The model under review builds one solid part; all positions refer to its coordinate system, in mm. Face numbers are marked on the shaded views. A direction names the side the tool comes from. Round coordinates to 2 decimals unless told otherwise and drop trailing zeros. Loops run counter-clockwise (first coordinate to the right, second up) from the corner with the lowest first, then second, coordinate; pieces in that order, holes last. Notation, with made-up numbers: (34.25, 73.25) -> (90.25, 73.25) arc R22 ccw to (90.25, 85.25) -> close; hole circle Ø9 at (36.5, 29). An arc over 180 degrees is marked (long way). Use a Markdown table: item, result. Add a question column.
1) Mouldability with a two-part tool opening along Y and no side actions: class the marked faces 1, 2 and 3 as released by +Y, released by -Y, zero draft, split by the parting line, or undercut.
2) Wall thickness on probe 1 along X at (y, z) = (-15.5, 5.5); probe 2 along X at (y, z) = (-9, 6.5); probe 3 along X at (y, z) = (10, 3.5): over which ranges is each line inside the solid? List them lowest first.
3) Insertion check: pin 1 (1 mm diameter, centred on x = -9.5, z = 1.5, fed in from -Y); pin 2 (2 mm diameter, centred on y = 23.5, z = 3, fed in from +X); pin 3 (6 mm diameter, centred on x = 11.14, y = 11.14, fed in from +Z); pin 4 (2 mm diameter, centred on x = -20.67, y = 7.52, fed in from +Z). Each pin has a flat end and moves straight along its axis. Give the tip position at first contact, or say it passes through.
4) Consider section A-A on z = 7. State how many separate pieces and enclosed holes the cut face has, plus the area to 3 significant figures.
5) For the marked faces 4 and 5, list the 3-axis set-ups (+Z, -Z, +X, -X, +Y, -Y) from which the entire face can be reached by the end or side of a thin tool; tool diameter is ignored.
6) Consider section B-B on y = 20. Give the boundary of the cut face in (x, z), plus the area to 3 significant figures.
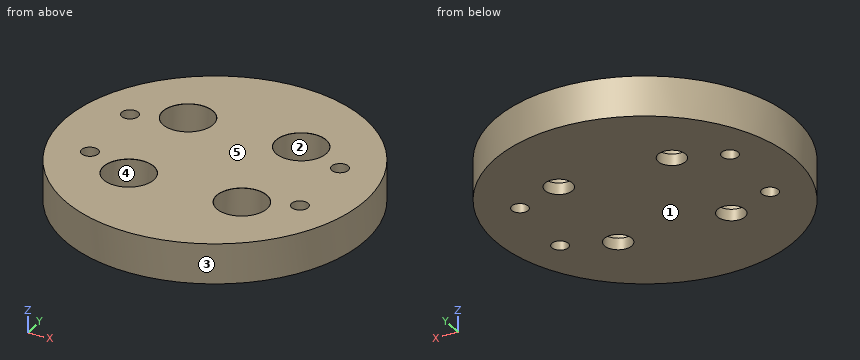
from build123d import *

# Parameters (mm, degrees)
SKETCH_1_R               = 30
EXTRUDE_1_DEPTH          = 8
PATTERN_CIRCULAR_1_COUNT = 4
HOLE_WIZARD_M4_1_D       = 3.3


with BuildPart() as part:
    # 草图1 → 凸台-拉伸1 (new body)
    with BuildSketch(Plane.XY):
        Circle(SKETCH_1_R)
    extrude(amount=EXTRUDE_1_DEPTH)

    # 草图7 → 打孔尺寸(%根据)内六角圆柱头螺钉的类型1 (revolve, cut)
    with BuildSketch(Plane(origin=(11.136931804, -11.136931804, 8), x_dir=(0, -1, 0), z_dir=(1, 0, 0))):
        Polygon((0, 0), (0, 8), (2.75, 8), (2.75, 5.7), (5, 5.7), (5, 0.025), (5.025, 0), align=None)
    hole_wizard_1 = revolve(axis=Axis((11.136931804, -11.136931804, 14.35), (0, 0, -1)), mode=Mode.SUBTRACT)

    # 阵列(圆周)1: 打孔尺寸(%根据)内六角圆柱头螺钉的类型1 ×4 about axis
    pattern_circular_1_axis = Axis((0, 0, 0), (0, 0, 1))
    for i in range(1, PATTERN_CIRCULAR_1_COUNT):
        add(hole_wizard_1.rotate(pattern_circular_1_axis, i * 360 / PATTERN_CIRCULAR_1_COUNT), mode=Mode.SUBTRACT)

    # M4 螺纹孔1 (through all)
    with Locations(Plane.XY.offset(8)):
        with Locations((20.673237657, 7.524443153), (20.673237657, -7.524443153), (-20.673237657, 7.524443153), (-20.673237657, -7.524443153)):
            Hole(HOLE_WIZARD_M4_1_D / 2)


solid = part.part
Result set:
| question | item | result |
|---|---|---|
| 1 | face 1 | zero draft |
| 1 | face 2 | undercut |
| 1 | face 3 | split by the parting line |
| 2 | probe 1 | -25.69 to -13.58, -8.69 to 8.69, 13.58 to 25.69 |
| 2 | probe 2 | -28.62 to -21.41, -19.93 to -15.66, -6.62 to 6.62, 15.66 to 19.93, 21.41 to 28.62 |
| 2 | probe 3 | -28.28 to -16.01, -6.27 to 6.27, 16.01 to 28.28 |
| 3 | pin 1 | y = -28.62 |
| 3 | pin 2 | x = 19.84 |
| 3 | pin 3 | z = 2.3 |
| 3 | pin 4 | through |
| 4 | separate pieces | 1 |
| 4 | enclosed holes | 8 |
| 4 | area | 2,480 mm2 |
| 5 | face 4 | +Z |
| 5 | face 5 | +Z, +X, -X, +Y, -Y |
| 6 | outline | (-22.36, 0) -> (22.36, 0) -> (22.36, 8) -> (-22.36, 8) -> close |
| 6 | area | 358 mm2 |
